Answer from the drawing. Dimensions are ordinates in mm from the lowest x, y and z of the part. A direction names the side the tool comes from. Give positions to 0.01 mm unless a question says otherwise; leave off trailing zeros. Loops run counter-clockwise (first coordinate to the right, second up) from the corner with the lowest first, then second, coordinate; pieces in that order, holes last.
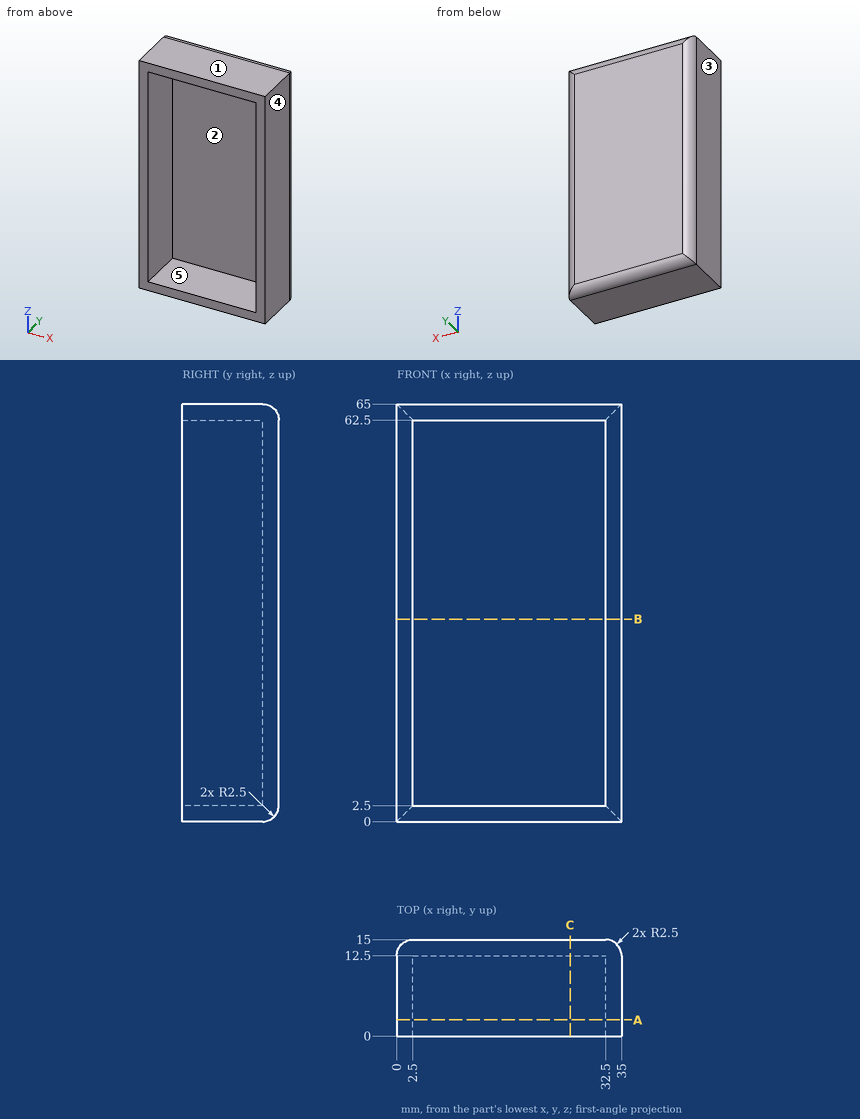
Item 1: Determine the mould class of the marked faces 3, 4 and 5 for opening direction X: released by +X, released by -X, zero draft, split by the parting line, or undercut.
Item 2: Find section C-C, the plane x = 27. Write down the section's boundary in (y, z).
Item 3: Find section A-A, the plane y = 2.5. Write down the section's boundary in (x, z).
Item 4: For the marked faces 1 and 2, determine the directions among +Z, -Z, +X, -X, +Y, -Y from which every point of the face is accessible in a straight line to the end or side of a thin tool.
Item 5: Consider line 1 (X direction, y = 7.75, z = 44); line 2 (Z direction, x = 24.5, y = 4); line 3 (Y direction, x = 11, z = 4). Determine where each line is inside the solid, lowest interval first.
Item 6: Find section B-B, the plane z = 31.5. Write down the section's boundary in (x, y), plus the area to 3 significant figures.
Ans:
1. face 3: released by -X
1. face 4: released by +X
1. face 5: undercut
2. outline: (0, 0) - (12.5, 0) arc R2.5 ccw to (15, 2.5) - (15, 62.5) arc R2.5 ccw to (12.5, 65) - (0, 65) - (0, 62.5) - (12.5, 62.5) - (12.5, 2.5) - (0, 2.5) - close
3. outline: (0, 0) - (35, 0) - (35, 65) - (0, 65) - close; hole (2.5, 2.5) - (32.5, 2.5) - (32.5, 62.5) - (2.5, 62.5) - close
4. face 1: +Z, +X, -X, +Y, -Y
4. face 2: -Y
5. line 1: x = 0 to 2.5, 32.5 to 35
5. line 2: z = 0 to 2.5, 62.5 to 65
5. line 3: y = 12.5 to 15
6. outline: (0, 0) - (2.5, 0) - (2.5, 12.5) - (32.5, 12.5) - (32.5, 0) - (35, 0) - (35, 12.5) arc R2.5 ccw to (32.5, 15) - (2.5, 15) arc R2.5 ccw to (0, 12.5) - close
6. area: 147 mm2
